The model under review builds one solid part; all positions refer to its coordinate system, in mm. A direction names the side the tool comes from. Give positions to 0.01 mm unless a question says otherwise; leave off trailing zeros. Order: outer loops, then holes, each group sorted by start corner. A loop starts at its lowest first (then second) coordinate and runs counter-clockwise, first axis right, second up. Notation, with made-up numbers: (54.25, 43.5) -> (65.25, 43.5) arc R18 cw to (65.25, 48.5) -> close; hole circle Ø6 at (87, 80.5). An arc over 180 degrees is marked (long way). Answer as a JSON object with one key per item and string values. Group by question number.
Autodesk Inventor part; units mm, degrees
ref_plane "YZ Plane" through (0, 0, 0) normal (1, 0, 0) x (0, 1, 0)
ref_plane "XZ Plane" through (0, 0, 0) normal (0, 1, 0) x (-1, 0, 0)
ref_plane "XY Plane" through (0, 0, 0) normal (0, 0, 1) x (1, 0, 0)
sketch "Sketch1" plane through (0, 0, 0) normal (0, 0, 1) x (1, 0, 0)
  line L0 (-5, -10.16) -> (5, -10.16)
  line L1 (5, -10.16) -> (5, 10.16)
  line L2 (5, 10.16) -> (-5, 10.16)
  line L3 (-5, 10.16) -> (-5, -10.16)
  line L4 (-5, -10.16) -> (5, 10.16) construction
  line L5 (5, -10.16) -> (-5, 10.16) construction
  line L6 (5, 10.16) -> (8.1852, 10.16)
  line L7 (8.1852, 10.16) -> (8.1852, -10.16)
  line L8 (8.1852, -10.16) -> (5, -10.16)
  line L9 (5, -10.16) -> (5, 10.16)
  line L10 (0, 10.16) -> (0, -10.16)
  line L11 (0, 10.16) -> (19.05, 10.16)
  line L12 (19.05, 10.16) -> (19.05, 13.335)
  line L13 (19.05, 13.335) -> (0, 13.335)
  line L14 (0, 13.335) -> (0, 10.16)
  line L15 (0, -10.16) -> (19.05, -10.16)
  line L16 (19.05, -10.16) -> (19.05, -13.335)
  line L17 (19.05, -13.335) -> (0, -13.335)
  line L18 (0, -13.335) -> (0, -10.16)
  point P0 (0, 0)
  point P1 (8.1852, -10.16)
  dimension "d0" = 10
  dimension "d1" = 20.32
  dimension "d2" = 3.1852
  dimension "d3" = 19.05
  dimension "d4" = 3.175
  dimension "d5" = 19.05
  dimension "d6" = 3.175
revolve "Revolution1" add sketch "Sketch1" angle 360 about axis through (0, 10.16, 0) along (0, -1, 0) contours L0 L8 L15 L16 L17 L18 | L1 L6 L7 L8 | L14 L13 L12 L11 L6 L2
sketch "Sketch2" plane through (0, 13.335, 0) normal (0, 1, 0) x (1, 0, 0)
  circle A0 centre (0, 0) radius 7
  line L0 (8, -8) -> (-8, -8)
  line L1 (-8, -8) -> (-8, 8)
  line L2 (-8, 8) -> (8, 8)
  line L3 (8, 8) -> (8, -8)
  line L4 (8, -8) -> (-8, 8) construction
  line L5 (-8, -8) -> (8, 8) construction
  circle A1 centre (-8, 8) radius 2.25
  circle A2 centre (8, 8) radius 2.25
  circle A3 centre (8, -8) radius 2.25
  circle A4 centre (-8, -8) radius 2.25
  dimension "d8" = 14
  dimension "d11" = 16
  dimension "d12" = 16
  dimension "d13" = 4.5
  dimension "d14" = 4.5
  dimension "d15" = 4.5
  dimension "d16" = 4.5
extrude "Extrusion1" cut sketch "Sketch2" against normal through all contours A0 | A4 L1 L0 | L0 L1 A4 | A3 L3 L0 | L0 L3 A3 | A1 L2 L1 | L1 L2 A1 | A2 L2 L3 | L3 L2 A2
properties part number "Slide_Climb_Spool"
1. Draft analysis for pull direction Y (two halves, no side actions). For faces 3 (the flat face through (8, -13.335, 0)), 4 (the cylindrical face through (-6.495, -0.142, -4.981)), 5 (the flat face through (8, 10.16, -4)), 6 (the cylindrical face through (6.34, 11.77, 6.48)), state which applies: pulls with the +Y half, pulls with the -Y half, needs draft (parallel to the pull), parting line crosses it, or undercut.
2. Take a section at B-B on x = 0. Give the boundary of the cut face in (y, z) (3 decimals), plus the area to 3 significant figures.
3. For pin 1 (18 mm diameter, centred on x = 0, z = 0, fed in from -Y) (3 decimals); pin 2 (8 mm diameter, centred on y = -2, z = -10, fed in from +X); pin 3 (8 mm diameter, centred on y = 9.5, z = -6.5, fed in from +X); pin 4 (6 mm diameter, centred on y = -10, z = 8.5, fed in from -X), all flat-tipped, find the tip position at first contact; note any pin that passes through.
4. Take a section at D-D on x = 6.5. State how many separate pieces and enclosed holes the cut face has, plus the area to 3 significant figures.
5. Machinability: for faces 1 (the cylindrical face through (-9.66, -11.73, -9.52)), 2 (the flat face through (8, -10.16, -4)), which of the approach directions +Z, -Z, +X, -X, +Y, -Y give a long, thin tool a straight path to every point of the face, cutting with its end or side? Answer none if there is none.
6. Take a section at C-C on y = 1.25. Give the boundary of the cut face in (x, z), plus the area to 3 significant figures.
7. Take a section at A-A on z = 0. Give the boundary of the cut face in (x, y) (3 decimals), plus the area to 3 significant figures.
8. For probe 1 along Z at (x, y) = (-8, -11.5); probe 2 along Y at (x, z) = (-13, 7.5) (3 decimals), list the stretches that pass through material, from the lowest coordinate up. Write a range as [from, to].
Checks:
{
 "1": {"face 3": "pulls with the -Y half", "face 4": "undercut", "face 5": "undercut", "face 6": "needs draft"},
 "2": {"outline": "(-13.335, -19.05) -> (-10.16, -19.05) -> (-10.16, -8.185) -> (10.16, -8.185) -> (10.16, -19.05) -> (13.335, -19.05) -> (13.335, -7) -> (-13.335, -7) -> close; (-13.335, 7) -> (13.335, 7) -> (13.335, 19.05) -> (10.16, 19.05) -> (10.16, 8.185) -> (-10.16, 8.185) -> (-10.16, 19.05) -> (-13.335, 19.05) -> close", "area": "201 mm2"},
 "3": {"pin 1": "stops at y = -13.335", "pin 2": "stops at x = 5.57", "pin 3": "stops at x = 18.88", "pin 4": "stops at x = -18.24"},
 "4": {"separate pieces": "6", "enclosed holes": "0", "area": "248 mm2"},
 "5": {"face 1": "+Y, -Y", "face 2": "none"},
 "6": {"outline": "circle Ø16.37 at (0, 0); hole circle Ø14 at (0, 0)", "area": "56.5 mm2"},
 "7": {"outline": "(-19.05, -13.335) -> (-7, -13.335) -> (-7, 13.335) -> (-19.05, 13.335) -> (-19.05, 10.16) -> (-8.185, 10.16) -> (-8.185, -10.16) -> (-19.05, -10.16) -> close; (7, -13.335) -> (19.05, -13.335) -> (19.05, -10.16) -> (8.185, -10.16) -> (8.185, 10.16) -> (19.05, 10.16) -> (19.05, 13.335) -> (7, 13.335) -> close", "area": "201 mm2"},
 "8": {"probe 1": "z = [-17.29, -10.25], [-5.75, 5.75], [10.25, 17.29]", "probe 2": "y = [-13.335, -10.16], [10.16, 13.335]"}
}
